from build123d import *

# Parameters (mm, degrees)
SKETCH005_W                               = 24
SKETCH005_H                               = 14
EXTRUDE006_DEPTH                          = 10
EXTRUDE007_DEPTH                          = 10
EXTRUDE005_DEPTH                          = 10
SKETCH004_W                               = 5
SKETCH004_H                               = 41
EXTRUDE004_DEPTH                          = 17
SKETCH003_AS_DRAWN_R                      = 1.5
EXTRUDE003_DEPTH                          = 5
EXTRUDE003_ONTO_SKETCH003_ROLL_ANGLE      = -90
EXTRUDE003_ONTO_SKETCH003_PITCH_ANGLE     = -89.903691
EXTRUDE003_ONTO_SKETCH003_PLACEMENT_ANGLE = -90
SKETCH002_W                               = 84
SKETCH002_H                               = 19
EXTRUDE002_DEPTH                          = 8
SKETCH001_W                               = 10
SKETCH001_H                               = 85
EXTRUDE001_DEPTH                          = 22.5
EXTRUDE_DEPTH                             = 90


with BuildPart() as extrude006:
    # Sketch005 (on Face18 of Fusion) → Extrude006 (new body)
    with BuildSketch(Plane(origin=(23, 0, 0), x_dir=(0, -1, 0), z_dir=(-1, 0, 0))):
        with Locations((-53.5, 42)):
            Rectangle(SKETCH005_W, SKETCH005_H)
        with BuildLine():
            add(Edge.make_bspline(
                [(-66.107143, 41.5), (-66.107143, 43.232051), (-68.946429, 42.366025), (-71.785714, 41.5), (-68.946429, 40.633975), (-66.107143, 39.767949), (-66.107143, 41.5)],
                knots=[0, 0, 0, 2.094395, 2.094395, 4.18879, 4.18879, 6.283185, 6.283185, 6.283185], degree=2, weights=[1, 0.5, 1, 0.5, 1, 0.5, 1]))
        make_face()
        with BuildLine():
            add(Edge.make_bspline(
                [(-37.107143, 41.5), (-37.107143, 43.232051), (-39.946429, 42.366025), (-42.785714, 41.5), (-39.946429, 40.633975), (-37.107143, 39.767949), (-37.107143, 41.5)],
                knots=[0, 0, 0, 2.094395, 2.094395, 4.18879, 4.18879, 6.283185, 6.283185, 6.283185], degree=2, weights=[1, 0.5, 1, 0.5, 1, 0.5, 1]))
        make_face()
    extrude(amount=-EXTRUDE006_DEPTH)


with BuildPart() as extrude007:
    # Sketch005 (on Face18 of Fusion) → Extrude007 (new body)
    with BuildSketch(Plane(origin=(23, 0, 0), x_dir=(0, -1, 0), z_dir=(-1, 0, 0))):
        with Locations((-53.5, 42)):
            Rectangle(SKETCH005_W, SKETCH005_H)
        with BuildLine():
            add(Edge.make_bspline(
                [(-66.107143, 41.5), (-66.107143, 43.232051), (-68.946429, 42.366025), (-71.785714, 41.5), (-68.946429, 40.633975), (-66.107143, 39.767949), (-66.107143, 41.5)],
                knots=[0, 0, 0, 2.094395, 2.094395, 4.18879, 4.18879, 6.283185, 6.283185, 6.283185], degree=2, weights=[1, 0.5, 1, 0.5, 1, 0.5, 1]))
        make_face()
        with BuildLine():
            add(Edge.make_bspline(
                [(-37.107143, 41.5), (-37.107143, 43.232051), (-39.946429, 42.366025), (-42.785714, 41.5), (-39.946429, 40.633975), (-37.107143, 39.767949), (-37.107143, 41.5)],
                knots=[0, 0, 0, 2.094395, 2.094395, 4.18879, 4.18879, 6.283185, 6.283185, 6.283185], degree=2, weights=[1, 0.5, 1, 0.5, 1, 0.5, 1]))
        make_face()
    extrude(amount=-EXTRUDE007_DEPTH)


with BuildPart() as motor_cavity:
    # Sketch005 (on Face18 of Fusion) → Extrude005 (new body)
    with BuildSketch(Plane(origin=(23, 0, 0), x_dir=(0, -1, 0), z_dir=(-1, 0, 0))):
        with Locations((-53.5, 42)):
            Rectangle(SKETCH005_W, SKETCH005_H)
        with BuildLine():
            add(Edge.make_bspline(
                [(-66.107143, 41.5), (-66.107143, 43.232051), (-68.946429, 42.366025), (-71.785714, 41.5), (-68.946429, 40.633975), (-66.107143, 39.767949), (-66.107143, 41.5)],
                knots=[0, 0, 0, 2.094395, 2.094395, 4.18879, 4.18879, 6.283185, 6.283185, 6.283185], degree=2, weights=[1, 0.5, 1, 0.5, 1, 0.5, 1]))
        make_face()
        with BuildLine():
            add(Edge.make_bspline(
                [(-37.107143, 41.5), (-37.107143, 43.232051), (-39.946429, 42.366025), (-42.785714, 41.5), (-39.946429, 40.633975), (-37.107143, 39.767949), (-37.107143, 41.5)],
                knots=[0, 0, 0, 2.094395, 2.094395, 4.18879, 4.18879, 6.283185, 6.283185, 6.283185], degree=2, weights=[1, 0.5, 1, 0.5, 1, 0.5, 1]))
        make_face()
    extrude(amount=-EXTRUDE005_DEPTH)

    # Fusion001: union Extrude006, Extrude007
    add(extrude006.part)
    add(extrude007.part)


with BuildPart() as motor_holder:
    # Sketch004 (on Face12 of Cut002) → Extrude004 (new body)
    with BuildSketch(Plane.XY.offset(35)):
        with Locations((25.5, 53)):
            Rectangle(SKETCH004_W, SKETCH004_H)
    extrude(amount=EXTRUDE004_DEPTH)


with BuildPart() as screw_holes:
    # Sketch003 as drawn → Extrude003 (new)
    with BuildSketch(Plane.XY):
        with Locations((16.786752, -38.744592)):
            Circle(SKETCH003_AS_DRAWN_R)
        with Locations((-18.213177, -38.677355)):
            Circle(SKETCH003_AS_DRAWN_R)
        with Locations((16.92963, 41.255274)):
            Circle(SKETCH003_AS_DRAWN_R)
        with Locations((-18.0703, 41.32251)):
            Circle(SKETCH003_AS_DRAWN_R)
    extrude(amount=-EXTRUDE003_DEPTH)


with BuildPart() as screw_holes_1:
    # Extrude003 onto Sketch003 roll: moved
    add(screw_holes.part.rotate(Axis((0, 0, 0), (1, 0, 0)), EXTRUDE003_ONTO_SKETCH003_ROLL_ANGLE))


with BuildPart() as screw_holes_2:
    # Extrude003 onto Sketch003 pitch: moved
    add(screw_holes_1.part.rotate(Axis((0, 0, 0), (0, 1, 0)), EXTRUDE003_ONTO_SKETCH003_PITCH_ANGLE))


with BuildPart() as screw_holes_3:
    # Extrude003 onto Sketch003 placement: moved
    add(screw_holes_2.part.moved(Location((3, 46.287879, 23.143939))).rotate(Axis((3, 46.287879, 23.143939), (0, 0, 1)), EXTRUDE003_ONTO_SKETCH003_PLACEMENT_ANGLE))


with BuildPart() as cavity:
    # Sketch002 (on Face8 of Cut) → Extrude002 (new body)
    with BuildSketch(Plane.YZ.offset(28)):
        with Locations((45, 22.5)):
            Rectangle(SKETCH002_W, SKETCH002_H)
    extrude(amount=-EXTRUDE002_DEPTH)


with BuildPart() as lock_hole:
    # Sketch001 (on Face4 of Extrude) → Extrude001 (new body)
    with BuildSketch(Plane.XY.offset(35)):
        with Locations((8, 47.5)):
            Rectangle(SKETCH001_W, SKETCH001_H)
    extrude(amount=-EXTRUDE001_DEPTH)


with BuildPart() as cut003:
    # Sketch → Extrude (new body)
    with BuildSketch(Plane.XZ):
        Polygon((0, 0), (0, 45), (3, 45), (3, 35), (28, 35), (28, 10), (3, 10), (3, 0), align=None)
    extrude(amount=-EXTRUDE_DEPTH)

    # Cut: cut lock hole
    add(lock_hole.part, mode=Mode.SUBTRACT)

    # Cut001: cut cavity
    add(cavity.part, mode=Mode.SUBTRACT)

    # Cut002: cut screw holes
    add(screw_holes_3.part, mode=Mode.SUBTRACT)

    # Fusion: union motor holder
    add(motor_holder.part)

    # Cut003: cut motor cavity
    add(motor_cavity.part, mode=Mode.SUBTRACT)


solid = cut003.part
Source: CAD feature listing. Evaluate the final solid. Frame: model axes, mm. A direction names the side the tool comes from. Coordinates: 2 decimals unless noted, no trailing zeros. Loops run counter-clockwise (first coordinate to the right, second up) from the corner with the lowest first, then second, coordinate; pieces in that order, holes last. Notation, with made-up numbers: (-38, -5.5) - (20, -5.5) arc R35 ccw to (20, 30.5) - close; hole circle Ø5 at (46, -23). An arc over 180 degrees is marked (long way). One line per item, written item: value. Start each with the question number.
1. Section A-A (z = 47). Return the cut outline in (x, y).
2. Contact query for flat-ended pins moving along their axis: P1, Ø6, axis at x = 17, y = 41.5, coming from the +Z side; P2, Ø1.5, axis at x = 21, y = 70.5, coming from the -Z side; P3, Ø2.5, axis at x = 26, z = 40, coming from the +Y side. Output: stop coordinate, or through.
3. Mould query, pull axis Y, two halves, no side actions, for faces 4 (the flat face through (8, 5, 24)), 5 (the flat face through (1, 44, 45)), 6 (the flat face through (25, 32.5, 43)), 7 (the flat face through (24, 3, 22)). Classes: pulls with the +Y half, pulls with the -Y half, needs draft (parallel to the pull), parting line crosses it, or undercut.
4. Set-up query: faces 1 (the flat face through (8, 48, 12.5)), 2 (the flat face through (25, 65.5, 42)), 3 (the flat face through (25, 54, 49)). Return all of +Z, -Z, +X, -X, +Y, -Y with unobstructed straight access to the full face (end or side cutting, diameter ignored); none if empty.
5. Section C-C (x = 21.5). Return the cut outline in (y, z).
6. Section B-B (y = 61). Return the cut outline in (x, z).
7. Section D-D (y = 20). Return the cut outline in (x, z).
8. Ray query, L1, parallel to X at y = 69.5, z = 43.5; L2, parallel to X at y = 32.5, z = 19.5; L3, parallel to Z at x = 27, y = 74.5. Return the intervals inside material, ascending.
Verdict:
1. outline: (23, 32.5) - (28, 32.5) - (28, 41.5) - (23, 41.5) - close; (23, 65.5) - (28, 65.5) - (28, 73.5) - (23, 73.5) - close
2. P1: stops at z = 35
2. P2: stops at z = 10
2. P3: stops at y = 73.5
3. face 4: pulls with the +Y half
3. face 5: needs draft
3. face 6: pulls with the -Y half
3. face 7: undercut
4. face 1: +Z, +Y
4. face 2: +X
4. face 3: +X, -X
5. outline: (0, 10) - (90, 10) - (90, 35) - (0, 35) - close; hole (3, 13) - (87, 13) - (87, 32) - (3, 32) - close
6. outline: (0, 0) - (3, 0) - (3, 10) - (28, 10) - (28, 13) - (20, 13) - (20, 32) - (28, 32) - (28, 35) - (13, 35) - (13, 12.5) - (3, 12.5) - (3, 45) - (0, 45) - close; (23, 49) - (28, 49) - (28, 52) - (23, 52) - close
7. outline: (0, 0) - (3, 0) - (3, 10) - (28, 10) - (28, 13) - (20, 13) - (20, 32) - (28, 32) - (28, 35) - (13, 35) - (13, 12.5) - (3, 12.5) - (3, 45) - (0, 45) - close
8. L1: x = 0 to 3, 23 to 28
8. L2: x = 0 to 3, 13 to 20
8. L3: z = 10 to 13, 32 to 35
